from build123d import *

# Parameters (mm, degrees)
SKETCH1_R           = 5.5
BOSS_EXTRUDE1_DEPTH = 3.4
SKETCH3_R           = 2.55
CUT_EXTRUDE1_DEPTH  = 45.994538027
SKETCH4_W           = 2
SKETCH4_H           = 14
CUT_EXTRUDE2_DEPTH  = 1.25


with BuildPart() as part:
    # Sketch1 → Boss-Extrude1 (new body)
    # profile 1 of 7: a face of its own
    with BuildSketch(Plane(origin=(0, 0, 0), x_dir=(1, 0, 0), z_dir=(0, 1, 0))):
        Polygon((7.875644347, -7), (7.875644347, 7), (2.124355653, 10.320508076), (-10, 3.320508076), (-10, -3.320508076), (2.124355653, -10.320508076), align=None)
        with Locations(Location((0, 0, 0), (0, 0, 270))):
            Circle(SKETCH1_R, mode=Mode.SUBTRACT)
    # profile 2 of 7: a face of its own
    with BuildSketch(Plane(origin=(0, 0, 0), x_dir=(1, 0, 0), z_dir=(0, 1, 0))):
        Polygon((7.875644347, -7), (20, 0), (7.875644347, 7), align=None)
    # profile 3 of 7: a face of its own
    with BuildSketch(Plane(origin=(0, 0, 0), x_dir=(1, 0, 0), z_dir=(0, 1, 0))):
        Polygon((7.875644347, 7), (20, 0), (7.875644347, -7), (32.124355653, -7), (32.124355653, 7), align=None)
    # profile 4 of 7: a face of its own
    with BuildSketch(Plane(origin=(0, 0, 0), x_dir=(1, 0, 0), z_dir=(0, 1, 0))):
        Polygon((-10, -17.320508076), (2.124355653, -10.320508076), (-10, -3.320508076), align=None)
    # profile 5 of 7: a face of its own
    with BuildSketch(Plane(origin=(0, 0, 0), x_dir=(1, 0, 0), z_dir=(0, 1, 0))):
        Polygon((-10, -31.320508076), (2.124355653, -10.320508076), (-10, -17.320508076), (-10, -3.320508076), (-22.124355653, -24.320508076), align=None)
    # profile 6 of 7: a face of its own
    with BuildSketch(Plane(origin=(0, 0, 0), x_dir=(1, 0, 0), z_dir=(0, 1, 0))):
        Polygon((-10, 3.320508076), (2.124355653, 10.320508076), (-10, 17.320508076), align=None)
    # profile 7 of 7: a face of its own
    with BuildSketch(Plane(origin=(0, 0, 0), x_dir=(1, 0, 0), z_dir=(0, 1, 0))):
        Polygon((-10, 17.320508076), (2.124355653, 10.320508076), (-10, 31.320508076), (-22.124355653, 24.320508076), (-10, 3.320508076), align=None)
    extrude(amount=BOSS_EXTRUDE1_DEPTH)

    # Sketch3 → Cut-Extrude1 (cut, through all)
    with BuildSketch(Plane(origin=(0, 3.4, 0), x_dir=(1, 0, 0), z_dir=(0, 1, 0))):
        with Locations(Location((28.124355653, 3.5, 0), (0, 0, 270))):
            Circle(SKETCH3_R)
        with Locations(Location((28.124355653, -3.5, 0), (0, 0, 90))):
            Circle(SKETCH3_R)
        with Locations(Location((-11.031088913, -26.106406461, 0), (0, 0, 270))):
            Circle(SKETCH3_R)
        with Locations(Location((-17.09326674, -22.606406461, 0), (0, 0, 90))):
            Circle(SKETCH3_R)
        with Locations(Location((-17.09326674, 22.606406461, 0), (0, 0, 270))):
            Circle(SKETCH3_R)
        with Locations(Location((-11.031088913, 26.106406461, 0), (0, 0, 90))):
            Circle(SKETCH3_R)
    extrude(amount=-CUT_EXTRUDE1_DEPTH, mode=Mode.SUBTRACT)

    # Sketch4 → Cut-Extrude2 (cut)
    with BuildSketch(Plane.XZ):
        with Locations((8.875644347, 0)):
            Rectangle(SKETCH4_W, SKETCH4_H)
        Polygon((-11, -5.052558883), (-10, -3.320508076), (2.124355653, -10.320508076), (1.124355653, -12.052558883), align=None)
        Polygon((1.124355653, 12.052558883), (2.124355653, 10.320508076), (-10, 3.320508076), (-11, 5.052558883), align=None)
    extrude(amount=-CUT_EXTRUDE2_DEPTH, mode=Mode.SUBTRACT)


solid = part.part
Part model, mm, in its own coordinate system. A direction names the side the tool comes from. Coordinates: 2 decimals unless noted, no trailing zeros. Order: outer loops, then holes, each group sorted by start corner. A loop starts at its lowest first (then second) coordinate and runs counter-clockwise, first axis right, second up.
(1) Tool access for faces 4 (the face through (-10, 2, 0)), 5 (the face through (-4, 1.25, -8)), 6 (the face through (-5.2, 0, -2.4)), 7 (the face through (20, 2, -7)), 8 (the face through (-3, 3.4, -5)): list every direction of +Z, -Z, +X, -X, +Y, -Y with a clear straight run to the whole face (end or side of a thin tool).
Check sheet entries:
face 4: -X, +Y, -Y
face 5: -Y
face 6: +Z, -Z, +X, -X, -Y
face 7: -Z, +X, +Y, -Y
face 8: +Z, -Z, +X, -X, +Y
(2) Probe L1, parallel to Z at x = -16, y = 1.6; L2, parallel to X at y = 1.3, z = 0; L3, parallel to Z at x = -15, y = 1.85. List the from-to ranges inside material, lowest first.
Check sheet entries:
L1: z = -27.86 to -24.91, -20.3 to -13.71, 13.71 to 20.3, 24.91 to 27.86
L2: x = -10 to -5.5, 5.5 to 32.12
L3: z = -28.43 to -24.06, -21.15 to -11.98, 11.98 to 21.15, 24.06 to 28.43
(3) Slice it at D-D, the plane z = -22. Write the cut outline in (x, y).
Check sheet entries:
outline: (-20.78, 0) - (-19.57, 0) - (-19.57, 3.4) - (-20.78, 3.4) - close; (-14.62, 0) - (-4.62, 0) - (-4.62, 3.4) - (-14.62, 3.4) - close
(4) Slice it at A-A, the plane z = 0. Write the cut outline in (x, y), and give its area (3 significant figures).
Check sheet entries:
outline: (-10, 0) - (-5.5, 0) - (-5.5, 3.4) - (-10, 3.4) - close; (5.5, 0) - (7.88, 0) - (7.88, 1.25) - (9.88, 1.25) - (9.88, 0) - (32.12, 0) - (32.12, 3.4) - (5.5, 3.4) - close
area: 103 mm2
(5) Pin check, flat tips, straight feed: pin 1 Ø1.5 at (x, y) = (10, 0.5) entering from -Z; pin 2 Ø14.5 at (x, z) = (0, 0) entering from +Y; pin 3 Ø1.7 at (x, y) = (24, 2) entering from +Z; pin 4 Ø1.4 at (y, z) = (0.5, 2) entering from -X. Stop position of each tip, or through.
Check sheet entries:
pin 1: stops at z = -7
pin 2: stops at y = 3.4
pin 3: stops at z = 7
pin 4: stops at x = -10
(6) Slice it at B-B, the plane x = 0. Write the cut outline in (y, z), and give its area (3 significant figures).
Check sheet entries:
outline: (0, -14) - (3.4, -14) - (3.4, -5.5) - (0, -5.5) - (0, -9.09) - (1.25, -9.09) - (1.25, -11.4) - (0, -11.4) - close; (0, 5.5) - (3.4, 5.5) - (3.4, 14) - (0, 14) - (0, 11.4) - (1.25, 11.4) - (1.25, 9.09) - (0, 9.09) - close
area: 52.0 mm2
(7) Pull direction Z, two halves, no side cores. Call faces 1 (the face through (-15.98, 1.68, -27.87)), 2 (the face through (9.876, 1, 0)), 3 (the face through (-12.755, 1.724, -24.227)): pulls with the +Z half, pulls with the -Z half, needs draft (parallel to the pull), parting line crosses it, or undercut.
Check sheet entries:
face 1: pulls with the -Z half
face 2: needs draft
face 3: undercut
(8) Slice it at C-C, the plane y = 2.75. Write the cut outline in (x, z).
Check sheet entries:
outline: (-22.12, -24.32) - (-10, -31.32) - (2.12, -10.32) - (7.88, -7) - (32.12, -7) - (32.12, 7) - (7.88, 7) - (2.12, 10.32) - (-10, 31.32) - (-22.12, 24.32) - (-10, 3.32) - (-10, -3.32) - close; hole circle Ø5.1 at (-17.09, -22.61); hole circle Ø5.1 at (-17.09, 22.61); hole circle Ø5.1 at (-11.03, -26.11); hole circle Ø5.1 at (-11.03, 26.11); hole circle Ø11 at (0, 0); hole circle Ø5.1 at (28.12, -3.5); hole circle Ø5.1 at (28.12, 3.5)
